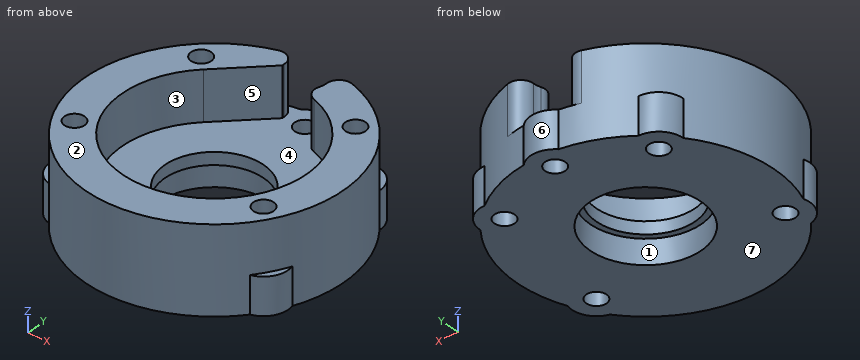
```python
from build123d import *

# Parameters (mm, degrees)
SKETCH_R        = 21
PAD_DEPTH       = 14
SKETCH001_R     = 9.05
POCKET_DEPTH    = 4
SKETCH002_R     = 8.05
POCKET001_DEPTH = 14.001
SKETCH003_R     = 15
POCKET002_DEPTH = 8.001
POCKET003_DEPTH = 8
SKETCH005_R     = 3.5
POCKET004_DEPTH = 8
FILLET_R        = 2
SKETCH006_R     = 4
PAD001_DEPTH    = 6
SKETCH007_R     = 1.65
POCKET005_DEPTH = 14.001


with BuildPart() as part:
    # Sketch → Pad (new body)
    with BuildSketch(Plane.XY):
        Circle(SKETCH_R)
    extrude(amount=PAD_DEPTH)

    # Sketch001 (on DatumPlane) → Pocket (cut)
    with BuildSketch(Plane.XY):
        Circle(SKETCH001_R)
    extrude(amount=POCKET_DEPTH, mode=Mode.SUBTRACT)

    # Sketch002 (on DatumPlane) → Pocket001 (cut, through all)
    with BuildSketch(Plane.XY):
        Circle(SKETCH002_R)
    extrude(amount=POCKET001_DEPTH, mode=Mode.SUBTRACT)

    # Sketch003 (on DatumPlane) → Pocket002 (cut, through all)
    with BuildSketch(Plane.XY.offset(6)):
        Circle(SKETCH003_R)
    extrude(amount=POCKET002_DEPTH, mode=Mode.SUBTRACT)

    # Sketch004 (on DatumPlane) → Pocket003 (cut)
    with BuildSketch(Plane.XY.offset(14)):
        Polygon((-10.606602, 10.606602), (0, 10.606602), (0, 21.213203), align=None)
    extrude(amount=-POCKET003_DEPTH, mode=Mode.SUBTRACT)

    # Sketch005 (on DatumPlane) → Pocket004 (cut)
    with BuildSketch(Plane.XY.offset(14)):
        with Locations((0, 18)):
            Circle(SKETCH005_R)
    extrude(amount=-POCKET004_DEPTH, mode=Mode.SUBTRACT)

    # Fillet
    fillet_edges = [part.edges().sort_by_distance(p)[0] for p in [
        (-1.945126, 20.909722, 10),
        (1.945126, 20.909722, 10),
        (1.643223, 14.909722, 10),
    ]]
    fillet(fillet_edges, radius=FILLET_R)

    # Sketch006 (on DatumPlane) → Pad001 (join)
    with BuildSketch(Plane.XY):
        with Locations((0, 18)):
            Circle(SKETCH006_R)
        with Locations((-12.727922, 12.727922)):
            Circle(SKETCH006_R)
        with Locations((12.727922, 12.727922)):
            Circle(SKETCH006_R)
        with Locations((-15.588457, -9)):
            Circle(SKETCH006_R)
        with Locations((15.588457, -9)):
            Circle(SKETCH006_R)
    extrude(amount=PAD001_DEPTH)

    # Sketch007 (on DatumPlane) → Pocket005 (cut, through all)
    with BuildSketch(Plane.XY):
        with Locations((-12.727922, 12.727922)):
            Circle(SKETCH007_R)
        with Locations((12.727922, 12.727922)):
            Circle(SKETCH007_R)
        with Locations((0, 18)):
            Circle(SKETCH007_R)
        with Locations((-15.588457, -9)):
            Circle(SKETCH007_R)
        with Locations((15.588457, -9)):
            Circle(SKETCH007_R)
    extrude(amount=POCKET005_DEPTH, mode=Mode.SUBTRACT)


solid = part.part
```
The listing builds one solid part. Answer for the finished solid, in the listing's coordinates (mm). Face numbers are marked on the shaded views. A direction names the side the tool comes from. Coordinates: 2 decimals unless noted, no trailing zeros. Write each loop counter-clockwise with the first axis right and the second up, starting at its lowest first coordinate (ties: lowest second). Pieces come first, ordered by that corner, then holes. Notation, with made-up numbers: (18, 80) - (76, 80) arc R25 ccw to (76, 93) - close; hole circle Ø7 at (-5.75, 89). An arc over 180 degrees is marked (long way). Return JSON: item names as keys, results as strings. Group by question number.
Q1. The part is cut by section B-B on y = 0. Write down the section's boundary in (x, z).
Q2. The part is cut by section C-C on y = -6.5. Write down the section's boundary in (x, z), and give its area (3 significant figures).
Q3. The part is cut by section A-A on x = 0. Write down the section's boundary in (y, z).
Q4. Find the intervals of material crossed by line 1 along X through (y, z) = (-9, 4.75); line 2 along Y through (x, z) = (0, 2.5); line 3 along X through (y, z) = (-9, 10.25), in increasing order. Write a range as [from, to].
Q5. Which of the six approach directions +Z, -Z, +X, -X, +Y, -Y give full straight-line access (tool end or side, diameter ignored) to the marked faces 1, 2 and 3?
Q6. The part is cut by section D-D on z = 12.25. State how many separate pieces and enclosed holes the cut face has, and give its area (3 significant figures).
Q7. For a pull along Y with two mould halves and no side action, classify the marked faces 4, 5, 6 and 7 as +Y half, -Y half, draft (parallel to the pull), parting line (faces both ways), or undercut.
Q8. Flat-ended cylindrical pins translate along their axes: pin 1 Ø9 at (x, y) = (-3.5, 11.5) entering from +Z; pin 2 Ø1.5 at (x, y) = (9.5, -1.5) entering from +Z; pin 3 Ø9.5 at (x, y) = (0, 0) entering from -Z; pin 4 Ø3 at (x, z) = (10.5, 7) entering from -Y. Find the tip coordinate at first contact, or state that the pin passes through.
Evaluation:
{
 "1": {"outline": "(-21, 0) - (-9.05, 0) - (-9.05, 4) - (-8.05, 4) - (-8.05, 6) - (-15, 6) - (-15, 14) - (-21, 14) - close; (8.05, 4) - (9.05, 4) - (9.05, 0) - (21, 0) - (21, 14) - (15, 14) - (15, 6) - (8.05, 6) - close"},
 "2": {"outline": "(-19.97, 0) - (-6.3, 0) - (-6.3, 4) - (-4.75, 4) - (-4.75, 6) - (-13.52, 6) - (-13.52, 14) - (-19.97, 14) - close; (4.75, 4) - (6.3, 4) - (6.3, 0) - (19.97, 0) - (19.97, 14) - (13.52, 14) - (13.52, 6) - (4.75, 6) - close", "area": "273 mm2"},
 "3": {"outline": "(-21, 0) - (-9.05, 0) - (-9.05, 4) - (-8.05, 4) - (-8.05, 6) - (-15, 6) - (-15, 14) - (-21, 14) - close; (8.05, 4) - (9.05, 4) - (9.05, 0) - (16.35, 0) - (16.35, 6) - (8.05, 6) - close; (19.65, 0) - (22, 0) - (22, 6) - (19.65, 6) - close"},
 "4": {"line 1": "x = [-19.59, -17.24], [-13.94, 13.94], [17.24, 19.59]", "line 2": "y = [-21, -9.05], [9.05, 16.35], [19.65, 22]", "line 3": "x = [-18.97, -17.24], [-13.94, -12], [12, 13.94], [17.24, 18.97]"},
 "5": {"face 1": "-Z", "face 2": "+Z, +X, -X, +Y, -Y", "face 3": "+Z"},
 "6": {"separate pieces": "1", "enclosed holes": "4", "area": "591 mm2"},
 "7": {"face 4": "undercut", "face 5": "undercut", "face 6": "+Y half", "face 7": "draft"},
 "8": {"pin 1": "stops at z = 14", "pin 2": "stops at z = 6", "pin 3": "passes through", "pin 4": "stops at y = -18.97"}
}
